Can you work these out from the model? Positions are in its coordinate system, mm. A direction names the side the tool comes from. Coordinates: 2 decimals unless noted, no trailing zeros. Loops run counter-clockwise (first coordinate to the right, second up) from the corner with the lowest first, then second, coordinate; pieces in that order, holes last. Notation, with made-up numbers: (83.25, 53.25) -> (135.25, 53.25) arc R26 ccw to (135.25, 92.25) -> close; hole circle Ø2 at (16.5, 61). An arc over 180 degrees is marked (long way). Put each result on its own line as item: value. Start each with the question number.
Item 1: Please list where these lines run through material, in increasing order: L1, parallel to X at y = 2.95, z = -17.5; L2, parallel to Z at x = 12.5, y = -0.5; L3, parallel to X at y = 3, z = 18. Write a range as from..to.
Item 2: We'd pull the mould along Z, two halves only. Please class faces 1 (the flat face through (-11.9, 5.8, -22)), 2 (the cylindrical face through (-28.479, 2.991, -16.345)), 3 (the flat face through (0, 6, -22.6)), 4 (the flat face through (-2.3, 7.9, -21.2)): pulls with the +Z half, pulls with the -Z half, needs draft (parallel to the pull), parting line crosses it, or undercut.
Item 3: For faces 5 (the flat face through (28, 0, -18)), 6 (the flat face through (32, 6, 13)), 7 (the flat face through (-25.5, 3, -18)), 8 (the flat face through (-32, 5, 14)), which set-ups out of +Z, -Z, +X, -X, +Y, -Y let a thin tool reach every point of the face, with its end or its side?
Item 4: Will these pins go through, and if not, where does the flat tip stop? P1, Ø0.8, axis at y = 4, z = -21.5, coming from the -X side; P2, Ø0.7, axis at y = 4, z = -22.5, coming from the -X side; P3, Ø0.7, axis at y = 3.5, z = -22, coming from the +X side.
Item 5: If we section it at C-C on x = 28: Please give me the cut outline in (y, z), plus the area to 3 significant figures.
Item 6: If we section it at D-D on z = 1: Please give me the cut outline in (x, y).
Item 7: If we section it at B-B on z = -17.5: Please give me the cut outline in (x, y), plus the area to 3 significant figures.
Item 8: If we section it at A-A on y = 6.75: Please give me the cut outline in (x, z).
```python
from build123d import *

# Parameters (mm, degrees)
SKETCH_1_W             = 63
SKETCH_1_H             = 42
EXTRUDE_298_DEPTH      = 1.6
SKETCH_2_W             = 42
SKETCH_2_H             = 30
CUT_EXTRUDE_670_DEPTH  = 0.8
SKETCH_4_W             = 1.6
SKETCH_4_H             = 42
EXTRUDE_914_DEPTH      = 9.5
SKETCH_5_W             = 6
SKETCH_5_H             = 6
EXTRUDE_1303_DEPTH     = 5.9
SKETCH_6_R             = 1.25
CUT_EXTRUDE_1636_DEPTH = 7.9
SKETCH_9_W             = 66.2
SKETCH_9_H             = 9.5
EXTRUDE_4_DEPTH        = 1.6
SKETCH_10_W            = 6
SKETCH_10_H            = 5
CUT_EXTRUDE_2759_DEPTH = 1
CUT_EXTRUDE_3267_REACH = 56.836
FILLET_4_R             = 1
FILLET_5_R             = 3
TF_REACH               = 70.894
CUT_EXTRUDE_1_REACH    = 70.894


with BuildPart() as part:
    # 草图1 → Extrude 298 (new body)
    with BuildSketch(Plane(origin=(0, 0, 0), x_dir=(1, 0, 0), z_dir=(0, 1, 0))):
        Rectangle(SKETCH_1_W, SKETCH_1_H)
    extrude(amount=-EXTRUDE_298_DEPTH)

    # 草图2 → Cut-Extrude 670 (cut)
    with BuildSketch(Plane(origin=(0, 0, 0), x_dir=(1, 0, 0), z_dir=(0, 1, 0))):
        with Locations((10.5, 0)):
            Rectangle(SKETCH_2_W, SKETCH_2_H)
    extrude(amount=-CUT_EXTRUDE_670_DEPTH, mode=Mode.SUBTRACT)

    # 草图4 → Extrude 914 (add)
    with BuildSketch(Plane(origin=(0, -1.6, 0), x_dir=(-1, 0, 0), z_dir=(0, -1, 0))):
        with Locations((-32.3, 0)):
            Rectangle(SKETCH_4_W, SKETCH_4_H)
        with Locations((32.3, 0)):
            Rectangle(SKETCH_4_W, SKETCH_4_H)
    extrude(amount=-EXTRUDE_914_DEPTH)

    # 草图5 → Extrude 1303 (add)
    with BuildSketch(Plane(origin=(0, 0, 0), x_dir=(1, 0, 0), z_dir=(0, 1, 0))):
        with Locations((-28.5, 18)):
            Rectangle(SKETCH_5_W, SKETCH_5_H)
        with Locations((28.5, 18)):
            Rectangle(SKETCH_5_W, SKETCH_5_H)
        with Locations((-28.5, -18)):
            Rectangle(SKETCH_5_W, SKETCH_5_H)
        with Locations((28.5, -18)):
            Rectangle(SKETCH_5_W, SKETCH_5_H)
    extrude(amount=EXTRUDE_1303_DEPTH)

    # 草图6 → Cut-Extrude 1636 (cut)
    with BuildSketch(Plane(origin=(0, 7.9, 0), x_dir=(1, 0, 0), z_dir=(0, 1, 0))):
        with Locations(Location((-28, 17.5, 0), (0, 0, 270))):
            Circle(SKETCH_6_R)
        with Locations(Location((28, 17.5, 0), (0, 0, 270))):
            Circle(SKETCH_6_R)
        with Locations(Location((28, -17.5, 0), (0, 0, 270))):
            Circle(SKETCH_6_R)
        with Locations(Location((-28, -17.5, 0), (0, 0, 270))):
            Circle(SKETCH_6_R)
    extrude(amount=-CUT_EXTRUDE_1636_DEPTH, mode=Mode.SUBTRACT)

    # 草图9 → 凸台-拉伸4 (add)
    with BuildSketch(Plane(origin=(0, 0, -21), x_dir=(-1, 0, 0), z_dir=(0, 0, -1))):
        with Locations((0, 3.15)):
            Rectangle(SKETCH_9_W, SKETCH_9_H)
    extrude(amount=EXTRUDE_4_DEPTH)

    # 草图10 → Cut-Extrude 2759 (cut)
    with BuildSketch(Plane.XY.offset(-21)):
        with Locations((20.5, 3.5)):
            Rectangle(SKETCH_10_W, SKETCH_10_H)
        with Locations((8.8, 3.5)):
            Rectangle(SKETCH_10_W, SKETCH_10_H)
        with Locations((1.9, 3.5)):
            Rectangle(SKETCH_10_W, SKETCH_10_H)
        with Locations((-5, 3.5)):
            Rectangle(SKETCH_10_W, SKETCH_10_H)
        with Locations((-11.9, 3.5)):
            Rectangle(SKETCH_10_W, SKETCH_10_H)
    extrude(amount=-CUT_EXTRUDE_2759_DEPTH, mode=Mode.SUBTRACT)

    # 草图12 → Cut-Extrude 3267 (cut, up to next)
    with BuildSketch(Plane.XY.offset(-22), mode=Mode.PRIVATE) as cut_extrude_3267_sk1:
        with BuildLine():
            Line((6.3, 2.5), (6.3, 4.5))
            ThreePointArc((6.3, 4.5), (6.592893219, 5.207106781), (7.3, 5.5))
            Line((7.3, 5.5), (10.3, 5.5))
            ThreePointArc((10.3, 5.5), (11.007106781, 5.207106781), (11.3, 4.5))
            Line((11.3, 4.5), (11.3, 2.5))
            ThreePointArc((11.3, 2.5), (11.007106781, 1.792893219), (10.3, 1.5))
            Line((10.3, 1.5), (7.3, 1.5))
            ThreePointArc((7.3, 1.5), (6.592893219, 1.792893219), (6.3, 2.5))
        make_face()
    cut_extrude_3267_tool1 = extrude(cut_extrude_3267_sk1.sketch, amount=-CUT_EXTRUDE_3267_REACH, mode=Mode.PRIVATE) & part.part
    # 草图12 → Cut-Extrude 3267 (cut, up to next)
    with BuildSketch(Plane.XY.offset(-22), mode=Mode.PRIVATE) as cut_extrude_3267_sk2:
        with BuildLine():
            Line((19, 1.5), (22, 1.5))
            ThreePointArc((22, 1.5), (22.707106781, 1.792893219), (23, 2.5))
            Line((23, 2.5), (23, 4.5))
            ThreePointArc((23, 4.5), (22.707106781, 5.207106781), (22, 5.5))
            Line((22, 5.5), (19, 5.5))
            ThreePointArc((19, 5.5), (18.292893219, 5.207106781), (18, 4.5))
            Line((18, 4.5), (18, 2.5))
            ThreePointArc((18, 2.5), (18.292893219, 1.792893219), (19, 1.5))
        make_face()
    cut_extrude_3267_tool2 = extrude(cut_extrude_3267_sk2.sketch, amount=-CUT_EXTRUDE_3267_REACH, mode=Mode.PRIVATE) & part.part
    # 草图12 → Cut-Extrude 3267 (cut, up to next)
    with BuildSketch(Plane.XY.offset(-22), mode=Mode.PRIVATE) as cut_extrude_3267_sk3:
        with BuildLine():
            Line((-0.6, 2.5), (-0.6, 4.5))
            ThreePointArc((-0.6, 4.5), (-0.307106781, 5.207106781), (0.4, 5.5))
            Line((0.4, 5.5), (3.4, 5.5))
            ThreePointArc((3.4, 5.5), (4.107106781, 5.207106781), (4.4, 4.5))
            Line((4.4, 4.5), (4.4, 2.5))
            ThreePointArc((4.4, 2.5), (4.107106781, 1.792893219), (3.4, 1.5))
            Line((3.4, 1.5), (0.4, 1.5))
            ThreePointArc((0.4, 1.5), (-0.307106781, 1.792893219), (-0.6, 2.5))
        make_face()
    cut_extrude_3267_tool3 = extrude(cut_extrude_3267_sk3.sketch, amount=-CUT_EXTRUDE_3267_REACH, mode=Mode.PRIVATE) & part.part
    # 草图12 → Cut-Extrude 3267 (cut, up to next)
    with BuildSketch(Plane.XY.offset(-22), mode=Mode.PRIVATE) as cut_extrude_3267_sk4:
        with BuildLine():
            Line((-7.5, 2.5), (-7.5, 4.5))
            ThreePointArc((-7.5, 4.5), (-7.207106781, 5.207106781), (-6.5, 5.5))
            Line((-6.5, 5.5), (-3.5, 5.5))
            ThreePointArc((-3.5, 5.5), (-2.792893219, 5.207106781), (-2.5, 4.5))
            Line((-2.5, 4.5), (-2.5, 2.5))
            ThreePointArc((-2.5, 2.5), (-2.792893219, 1.792893219), (-3.5, 1.5))
            Line((-3.5, 1.5), (-6.5, 1.5))
            ThreePointArc((-6.5, 1.5), (-7.207106781, 1.792893219), (-7.5, 2.5))
        make_face()
    cut_extrude_3267_tool4 = extrude(cut_extrude_3267_sk4.sketch, amount=-CUT_EXTRUDE_3267_REACH, mode=Mode.PRIVATE) & part.part
    # 草图12 → Cut-Extrude 3267 (cut, up to next)
    with BuildSketch(Plane.XY.offset(-22), mode=Mode.PRIVATE) as cut_extrude_3267_sk5:
        with BuildLine():
            Line((-14.4, 2.5), (-14.4, 4.5))
            ThreePointArc((-14.4, 4.5), (-14.107106781, 5.207106781), (-13.4, 5.5))
            Line((-13.4, 5.5), (-10.4, 5.5))
            ThreePointArc((-10.4, 5.5), (-9.692893219, 5.207106781), (-9.4, 4.5))
            Line((-9.4, 4.5), (-9.4, 2.5))
            ThreePointArc((-9.4, 2.5), (-9.692893219, 1.792893219), (-10.4, 1.5))
            Line((-10.4, 1.5), (-13.4, 1.5))
            ThreePointArc((-13.4, 1.5), (-14.107106781, 1.792893219), (-14.4, 2.5))
        make_face()
    cut_extrude_3267_tool5 = extrude(cut_extrude_3267_sk5.sketch, amount=-CUT_EXTRUDE_3267_REACH, mode=Mode.PRIVATE) & part.part
    add(cut_extrude_3267_tool1.solids().sort_by_distance((8.8, 3.5, -22))[0], mode=Mode.SUBTRACT)
    add(cut_extrude_3267_tool2.solids().sort_by_distance((20.5, 3.5, -22))[0], mode=Mode.SUBTRACT)
    add(cut_extrude_3267_tool3.solids().sort_by_distance((1.9, 3.5, -22))[0], mode=Mode.SUBTRACT)
    add(cut_extrude_3267_tool4.solids().sort_by_distance((-5, 3.5, -22))[0], mode=Mode.SUBTRACT)
    add(cut_extrude_3267_tool5.solids().sort_by_distance((-11.9, 3.5, -22))[0], mode=Mode.SUBTRACT)

    # 圆角4
    fillet_4_edges = [part.edges().sort_by_distance(p)[0] for p in [
        (0, -1.6, -22.6),
        (33.1, -1.6, -0.8),
        (-33.1, -1.6, -0.8),
    ]]
    fillet(fillet_4_edges, radius=FILLET_4_R)

    # 圆角5
    # the kernel refuses this fillet: 3 mm, written as the material it takes off along each edge
    with BuildSketch(Plane(origin=(30.1, -1.6, -19.6), x_dir=(0, 0, -1), z_dir=(-1, 0, 0))) as fillet_5_piece_1:
        with BuildLine():
            CenterArc((2, -1), 1, 0, 90)
            Line((3, -1), (3, 0))
            Line((3, 0), (2, 0))
        make_face()
    revolve(axis=Axis((30.1, -1.6, -19.6), (0, -1, 0)), revolution_arc=90, mode=Mode.SUBTRACT)
    with BuildSketch(Plane(origin=(-30.1, -1.6, -19.6), x_dir=(-1, 0, 0), z_dir=(0, 0, 1))) as fillet_5_piece_2:
        with BuildLine():
            CenterArc((2, -1), 1, 0, 90)
            Line((3, -1), (3, 0))
            Line((3, 0), (2, 0))
        make_face()
    revolve(axis=Axis((-30.1, -1.6, -19.6), (0, -1, 0)), revolution_arc=90, mode=Mode.SUBTRACT)
    with BuildSketch(Plane(origin=(33.1, 15.4, -22.6), x_dir=(0, 0, 1), z_dir=(0, -1, 0)), Plane(origin=(-33.1, -1.6, -22.6), x_dir=(0, 0, 1), z_dir=(0, 1, 0))) as fillet_5_piece_3:
        with BuildLine():
            CenterArc((FILLET_5_R, FILLET_5_R), FILLET_5_R, 180, 90)
            Line((0, FILLET_5_R), (0, 0))
            Line((0, 0), (FILLET_5_R, 0))
        make_face()
    extrude(amount=17, mode=Mode.SUBTRACT)

    # 草图16 → tf (cut, up to next)
    with BuildSketch(Plane(origin=(-31.5, 0, 0), x_dir=(0, 0, -1), z_dir=(1, 0, 0)), mode=Mode.PRIVATE) as tf_sk1:
        with BuildLine():
            Line((-14, 7.9), (-2, 7.9))
            Line((-2, 7.9), (-2, 2.9))
            ThreePointArc((-2, 2.9), (-2.292893219, 2.192893219), (-3, 1.9))
            Line((-3, 1.9), (-13, 1.9))
            ThreePointArc((-13, 1.9), (-13.707106781, 2.192893219), (-14, 2.9))
            Line((-14, 2.9), (-14, 7.9))
        make_face()
    tf_tool1 = extrude(tf_sk1.sketch, amount=-TF_REACH, mode=Mode.PRIVATE) & part.part
    add(tf_tool1.solids().sort_by_distance((-31.5, 4.916651, 8))[0], mode=Mode.SUBTRACT)

    # 草图17 → 切除-拉伸1 (cut, up to next)
    with BuildSketch(Plane.ZY.offset(-31.5), mode=Mode.PRIVATE) as cut_extrude_1_sk1:
        with BuildLine():
            Line((7, 7.9), (13, 7.9))
            Line((13, 7.9), (13, 3.9))
            ThreePointArc((13, 3.9), (12.414213562, 2.485786438), (11, 1.9))
            Line((11, 1.9), (9, 1.9))
            ThreePointArc((9, 1.9), (7.585786438, 2.485786438), (7, 3.9))
            Line((7, 3.9), (7, 7.9))
        make_face()
    cut_extrude_1_tool1 = extrude(cut_extrude_1_sk1.sketch, amount=-CUT_EXTRUDE_1_REACH, mode=Mode.PRIVATE) & part.part
    # 草图17 → 切除-拉伸1 (cut, up to next)
    with BuildSketch(Plane.ZY.offset(-31.5), mode=Mode.PRIVATE) as cut_extrude_1_sk2:
        with BuildLine():
            Line((4, 7.9), (-6, 7.9))
            Line((-6, 7.9), (-6, 4.9))
            ThreePointArc((-6, 4.9), (-5.707106781, 4.192893219), (-5, 3.9))
            Line((-5, 3.9), (3, 3.9))
            ThreePointArc((3, 3.9), (3.707106781, 4.192893219), (4, 4.9))
            Line((4, 4.9), (4, 7.9))
        make_face()
    cut_extrude_1_tool2 = extrude(cut_extrude_1_sk2.sketch, amount=-CUT_EXTRUDE_1_REACH, mode=Mode.PRIVATE) & part.part
    add(cut_extrude_1_tool1.solids().sort_by_distance((31.5, 5.027861, 10))[0], mode=Mode.SUBTRACT)
    add(cut_extrude_1_tool2.solids().sort_by_distance((31.5, 5.91927, -1))[0], mode=Mode.SUBTRACT)


solid = part.part
```
Solutions:
1. L1: -33.1..-29.25, -26.75..-25.5, 25.5..26.75, 29.25..33.1
1. L2: -22.6..-15, 15..21
1. L3: -33.1..-29.15, -26.85..-25.5, 25.5..26.85, 29.15..33.1
2. face 1: pulls with the +Z half
2. face 2: undercut
2. face 3: pulls with the -Z half
2. face 4: needs draft
3. face 5: +Y
3. face 6: +X, -X, +Y
3. face 7: +Z, +Y
3. face 8: -X, +Y
4. P1: x = -32.7
4. P2: x = -31.68
4. P3: x = 32.29
5. outline: (-1.6, -21.6) arc R1 ccw to (-0.6, -22.6) -> (7.9, -22.6) -> (7.9, -21) -> (5.9, -21) -> (5.9, -18.75) -> (0, -18.75) -> (0, -16.25) -> (5.9, -16.25) -> (5.9, -15) -> (-0.8, -15) -> (-0.8, 15) -> (5.9, 15) -> (5.9, 16.25) -> (0, 16.25) -> (0, 18.75) -> (5.9, 18.75) -> (5.9, 21) -> (-1.6, 21) -> close
5. area: 99.5 mm^2
6. outline: (-33.1, -0.6) arc R1 ccw to (-32.1, -1.6) -> (32.1, -1.6) arc R1 ccw to (33.1, -0.6) -> (33.1, 3.9) -> (31.5, 3.9) -> (31.5, -0.8) -> (-10.5, -0.8) -> (-10.5, 0) -> (-31.5, 0) -> (-31.5, 7.9) -> (-33.1, 7.9) -> close
7. outline: (-33.1, -0.6) arc R1 ccw to (-32.1, -1.6) -> (32.1, -1.6) arc R1 ccw to (33.1, -0.6) -> (33.1, 7.9) -> (31.5, 7.9) -> (31.5, 5.9) -> (29.25, 5.9) -> (29.25, 0) -> (26.75, 0) -> (26.75, 5.9) -> (25.5, 5.9) -> (25.5, 0) -> (-25.5, 0) -> (-25.5, 5.9) -> (-26.75, 5.9) -> (-26.75, 0) -> (-29.25, 0) -> (-29.25, 5.9) -> (-31.5, 5.9) -> (-31.5, 7.9) -> (-33.1, 7.9) -> close
7. area: 172 mm^2
8. outline: (-33.1, -19.6) arc R3 ccw to (-30.1, -22.6) -> (30.1, -22.6) arc R3 ccw to (33.1, -19.6) -> (33.1, -6) -> (31.5, -6) -> (31.5, -21) -> (-31.5, -21) -> (-31.5, 2) -> (-33.1, 2) -> close; (-33.1, 14) -> (-31.5, 14) -> (-31.5, 21) -> (-33.1, 21) -> close; (31.5, 4) -> (33.1, 4) -> (33.1, 7) -> (31.5, 7) -> close; (31.5, 13) -> (33.1, 13) -> (33.1, 21) -> (31.5, 21) -> close
